Check sheet for the modelled part. Datum: model origin and axes. Units: mm. Face numbers are marked on the shaded views. A direction names the side the tool comes from. Give positions to 0.01 mm unless a question says otherwise; leave off trailing zeros. Write each loop counter-clockwise with the first axis right and the second up, starting at its lowest first coordinate (ties: lowest second). Pieces come first, ordered by that corner, then holes. Notation, with made-up numbers: (-13.75, 39) -> (-3.75, 39) arc R16 ccw to (-3.75, 61) -> close; hole circle Ø7 at (23.25, -32). An arc over 180 degrees is marked (long way). Return JSON: item names as keys, results as strings.
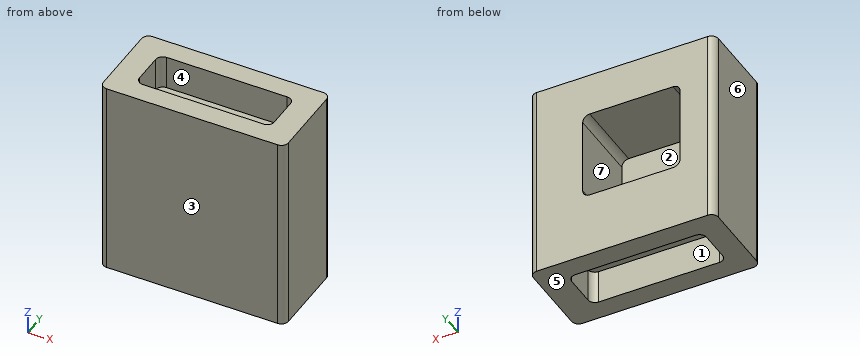
Autodesk Inventor part; units mm, degrees
ref_plane "YZ Plane" through (0, 0, 0) normal (1, 0, 0) x (0, 1, 0)
ref_plane "XZ Plane" through (0, 0, 0) normal (0, 1, 0) x (-1, 0, 0)
ref_plane "XY Plane" through (0, 0, 0) normal (0, 0, 1) x (1, 0, 0)
sketch "Sketch1" plane through (0, 0, 0) normal (0, 0, 1) x (1, 0, 0)
  line L0 (3.175, 0) -> (80.518, 0)
  line L1 (83.693, 3.175) -> (83.693, 35.433)
  line L2 (80.518, 38.608) -> (3.175, 38.608)
  line L3 (0, 35.433) -> (0, 3.175)
  arc A0 (3.175, 38.608) -> (0, 35.433) centre (3.175, 35.433) ccw
  arc A1 (0, 3.175) -> (3.175, 0) centre (3.175, 3.175) ccw
  arc A2 (80.518, 0) -> (83.693, 3.175) centre (80.518, 3.175) ccw
  arc A3 (83.693, 35.433) -> (80.518, 38.608) centre (80.518, 35.433) ccw
  point P0 (0, 0)
  point P1 (83.693, 38.608)
  point P2 (83.693, 0)
  point P3 (0, 38.608)
  dimension "d0" = 83.693
  dimension "d1" = 38.608
  dimension "d2" = 3.175
extrude "Extrusion1" add sketch "Sketch1" along normal blind 90.043
sketch "Sketch2" plane through (3.175, 38.608, 0) normal (0, 1, 0) x (1, 0, 0)
  line L0 (0, 0) -> (77.343, 0)
  line L1 (12.4957, 0) -> (42.2137, 0) construction
  line L2 (0, 0) -> (0, -90.043)
  line L3 (77.343, -90.043) -> (0, -90.043)
  line L4 (77.343, 0) -> (77.343, -90.043)
  line L5 (0, 0) -> (77.343, 0)
  line L6 (0, 0) -> (-3.175, 0)
  line L7 (80.518, 0) -> (77.343, 0)
  line L8 (-3.175, -90.043) -> (0, -90.043)
  line L9 (77.343, -90.043) -> (80.518, -90.043)
  line L10 (-3.175, 0) -> (-3.175, -90.043)
  line L11 (15.621, -29.718) -> (53.34, -29.718)
  line L12 (56.515, -32.893) -> (56.515, -67.31)
  line L13 (53.34, -70.485) -> (15.621, -70.485)
  line L14 (12.446, -67.31) -> (12.446, -32.893)
  arc A0 (15.621, -29.718) -> (12.446, -32.893) centre (15.621, -32.893) ccw
  arc A1 (56.515, -32.893) -> (53.34, -29.718) centre (53.34, -32.893) ccw
  arc A2 (53.34, -70.485) -> (56.515, -67.31) centre (53.34, -67.31) ccw
  arc A3 (12.446, -67.31) -> (15.621, -70.485) centre (15.621, -67.31) ccw
  point P0 (56.515, -70.485)
  point P1 (56.515, -29.718)
  point P2 (12.446, -70.485)
  dimension "d9" = 44.069
  dimension "d10" = 40.767
  dimension "d11" = 15.621
  dimension "d12" = 29.718
  dimension "d13" = 3.175
extrude "Extrusion2" cut sketch "Sketch2" against normal blind 33.02 contours L11 A1 L12 A2 L13 A3 L14 A0
sketch "Sketch3" plane through (0, 0, 90.043) normal (0, 0, 1) x (1, 0, 0)
  line L0 (80.518, 38.608) -> (3.175, 38.608)
  line L1 (11.684, 38.608) -> (20.955, 38.608) construction
  line L2 (14.5415, 29.337) -> (69.1515, 29.337)
  line L3 (72.3265, 26.162) -> (72.3265, 12.446)
  line L4 (69.1515, 9.271) -> (14.5415, 9.271)
  line L5 (11.3665, 12.446) -> (11.3665, 26.162)
  arc A0 (14.5415, 29.337) -> (11.3665, 26.162) centre (14.5415, 26.162) ccw
  arc A1 (72.3265, 26.162) -> (69.1515, 29.337) centre (69.1515, 26.162) ccw
  arc A2 (69.1515, 9.271) -> (72.3265, 12.446) centre (69.1515, 12.446) ccw
  arc A3 (11.3665, 12.446) -> (14.5415, 9.271) centre (14.5415, 12.446) ccw
  line L6 (83.693, 3.175) -> (83.693, 35.433)
  line L7 (0, 35.433) -> (0, 3.175)
  line L8 (3.175, 0) -> (80.518, 0)
  point P0 (0, 0)
  point P1 (72.3265, 9.271)
  point P2 (72.3265, 29.337)
  point P3 (11.3665, 9.271)
  dimension "d19" = 60.96
  dimension "d20" = 20.066
  dimension "d21" = 3.175
  dimension "d24" = 11.3665
  dimension "d25" = 9.271
extrude "Extrusion3" cut sketch "Sketch3" against normal blind 15.24
sketch "Sketch4" plane through (0, 0, 0) normal (0, 0, -1) x (-1, 0, 0)
  line L0 (-68.1482, 29.337) -> (-13.5382, 29.337)
  line L1 (-10.3632, 26.162) -> (-10.3632, 12.446)
  line L2 (-13.5382, 9.271) -> (-68.1482, 9.271)
  line L3 (-71.3232, 12.446) -> (-71.3232, 26.162)
  arc A0 (-68.1482, 29.337) -> (-71.3232, 26.162) centre (-68.1482, 26.162) ccw
  arc A1 (-10.3632, 26.162) -> (-13.5382, 29.337) centre (-13.5382, 26.162) ccw
  arc A2 (-13.5382, 9.271) -> (-10.3632, 12.446) centre (-13.5382, 12.446) ccw
  arc A3 (-71.3232, 12.446) -> (-68.1482, 9.271) centre (-68.1482, 12.446) ccw
  line L4 (-3.175, 38.608) -> (-80.518, 38.608)
  arc A4 (-80.518, 38.608) -> (-83.693, 35.433) centre (-80.518, 35.433) ccw
  line L5 (-83.693, 35.433) -> (-83.693, 3.175)
  arc A5 (-83.693, 3.175) -> (-80.518, 0) centre (-80.518, 3.175) ccw
  line L6 (-80.518, 0) -> (-3.175, 0)
  arc A6 (-3.175, 0) -> (0, 3.175) centre (-3.175, 3.175) ccw
  line L7 (0, 3.175) -> (0, 35.433)
  arc A7 (0, 35.433) -> (-3.175, 38.608) centre (-3.175, 35.433) ccw
  point P0 (0, 0)
  point P1 (-10.3632, 9.271)
  point P2 (-10.3632, 29.337)
  point P3 (-71.3232, 9.271)
  dimension "d28" = 60.96
  dimension "d29" = 20.066
  dimension "d30" = 3.175
  dimension "d31" = 10.3632
  dimension "d32" = 9.271
extrude "Extrusion5" cut sketch "Sketch4" against normal blind 15.24 contours L0 A1 L1 A2 L2 A3 L3 A0
properties part number "Middle Body"
(1) Depth check by flat-ended pin: pin 1 Ø10 at (x, y) = (29, 20) entering from +Z; pin 2 Ø12 at (x, z) = (38.5, 47) entering from +Y; pin 3 Ø3 at (x, y) = (16, 23) entering from -Z. Enter the tip coordinate at first touch or a pass-through.
Reply:
{"pin 1": "z = 74.8", "pin 2": "y = 5.59", "pin 3": "z = 15.24"}
(2) Thickness scan on L1, parallel to X at y = 20.5, z = 10; L2, parallel to Z at x = 19.5, y = 25.5 (3 decimals); L3, parallel to Y at x = 21.5, z = 85. Record the ranges inside material, lowest first.
Reply:
{"L1": "0 to 10.36, 71.32 to 83.69", "L2": "15.24 to 29.718, 70.485 to 74.803", "L3": "0 to 9.27, 29.34 to 38.61"}
(3) Cross-section at D-D on x = 64.5. Enter the section's corners in (y, z).
Reply:
{"outline": "(0, 0) -> (9.27, 0) -> (9.27, 15.24) -> (29.34, 15.24) -> (29.34, 0) -> (38.61, 0) -> (38.61, 90.04) -> (29.34, 90.04) -> (29.34, 74.8) -> (9.27, 74.8) -> (9.27, 90.04) -> (0, 90.04) -> close"}
(4) Cross-section at C-C on z = 55. Enter the section's corners in (x, y) (3 decimals), then the cut area to 3 significant figures.
Reply:
{"outline": "(0, 3.175) arc R3.175 ccw to (3.175, 0) -> (80.518, 0) arc R3.175 ccw to (83.693, 3.175) -> (83.693, 35.433) arc R3.175 ccw to (80.518, 38.608) -> (59.69, 38.608) -> (59.69, 5.588) -> (15.621, 5.588) -> (15.621, 38.608) -> (3.175, 38.608) arc R3.175 ccw to (0, 35.433) -> close", "area": "1,770 mm^2"}
(5) Set-up check for the marked faces 1, 2 and 3: record each of +Z, -Z, +X, -X, +Y, -Y from which the full face is reachable in a straight line by a thin tool's end or side.
Reply:
{"face 1": "-Z", "face 2": "+Y", "face 3": "+Z, -Z, +X, -X, -Y"}
(6) Release check for a two-part mould opening along X. For the marked faces 4, 5, 6 and 7 record: pulls with the +X half, pulls with the -X half, needs draft (parallel to the pull), parting line crosses it, or undercut.
Reply:
{"face 4": "undercut", "face 5": "needs draft", "face 6": "pulls with the -X half", "face 7": "undercut"}
(7) Cross-section at B-B on x = 45. Enter the section's corners in (y, z) (3 decimals).
Reply:
{"outline": "(0, 0) -> (9.271, 0) -> (9.271, 15.24) -> (29.337, 15.24) -> (29.337, 0) -> (38.608, 0) -> (38.608, 29.718) -> (5.588, 29.718) -> (5.588, 70.485) -> (38.608, 70.485) -> (38.608, 90.043) -> (29.337, 90.043) -> (29.337, 74.803) -> (9.271, 74.803) -> (9.271, 90.043) -> (0, 90.043) -> close"}
